CAD build for the part. Positions are in the model's coordinates, mm. A direction names the side the tool comes from. Give positions to 0.01 mm unless a question says otherwise; leave off trailing zeros. Loops run counter-clockwise (first coordinate to the right, second up) from the corner with the lowest first, then second, coordinate; pieces in that order, holes last. Notation, with made-up numbers: (-40, 48.5) -> (10, 48.5) arc R22 cw to (10, 66.5) -> close; hole circle Ø2 at (14, 56). An arc over 180 degrees is marked (long way). Use one line per item in the form item = value.
```python
from build123d import *

# Parameters (mm, degrees)
F0_R      = 15
F1_DEPTH  = 125
F2_W      = 15
F2_H      = 15
F3_ANGLE  = 90
F5_W      = 15
F5_H      = 15
F6_DEPTH  = 75
F8_R      = 5
F9_DEPTH  = 122.5
F10_R     = 5
F11_DEPTH = 122.5


with BuildPart() as f1:
    # F0 (on Right) → F1 (new body, symmetric)
    with BuildSketch(Plane.YZ):
        Circle(F0_R)
    extrude(amount=F1_DEPTH, both=True)

    # F4: F3 across plane


with BuildPart() as f3:
    # F2 (on face) → F3 (revolve)
    with BuildSketch(Plane.YZ.offset(125)):
        Rectangle(F2_W, F2_H)
    revolve(axis=Axis((125, 7.5, 0), (0, 0, 1)), revolution_arc=F3_ANGLE)


with BuildPart() as f1_1:
    add(f1.part)
    add(f3.part.mirror(Plane.YZ))


    add(f3.part)  # F6 merges F3
    # F5 (on face) → F6 (join)
    with BuildSketch(Plane(origin=(0, 7.5, 0), x_dir=(-1, 0, 0), z_dir=(0, 1, 0))):
        with Locations((-132.5, 0)):
            Rectangle(F5_W, F5_H)
    extrude(amount=F6_DEPTH)

    # F7: F1 across plane


with BuildPart() as f1_2:
    add(f1_1.part)
    add(f1_1.part.mirror(Plane.YZ))

    # F8 (on face) → F9 (join)
    with BuildSketch(Plane(origin=(-140, 0, 0), x_dir=(0, -1, 0), z_dir=(-1, 0, 0))):
        with Locations((-70, 0)):
            Circle(F8_R)
    extrude(amount=-F9_DEPTH)

    # F10 (on face) → F11 (join)
    with BuildSketch(Plane.YZ.offset(140)):
        with Locations((70, 0)):
            Circle(F10_R)
    extrude(amount=-F11_DEPTH)


solid = f1_2.part
```
1. Cut at D-D, the plane y = 70. Write the cut outline in (x, z).
Result sheet:
outline = (-140, -7.5) -> (-125, -7.5) -> (-125, -5) -> (-17.5, -5) -> (-17.5, 5) -> (-125, 5) -> (-125, 7.5) -> (-140, 7.5) -> close; (17.5, -5) -> (125, -5) -> (125, -7.5) -> (140, -7.5) -> (140, 7.5) -> (125, 7.5) -> (125, 5) -> (17.5, 5) -> close
2. Drop flat-ended pins along their axis: P1, Ø3, axis at x = 62.5, y = 9.5, coming from the -Z side; P2, Ø2, axis at x = -99, z = 10, coming from the -Y side; P3, Ø12, axis at x = 73.5, z = 5.5, coming from the +Y side. Give the stop position or say it passes through.
Result sheet:
P1 = -12.69
P2 = -12
P3 = 75
3. Tool access for faces 1 (the flat face through (17.5, 70, 0)), 2 (the flat face through (133, 37, -7.5)), 3 (the flat face through (-133, 37, 7.5)), 4 (the cylindrical face through (-72.002, 65.381, -1.915)): list every direction of +Z, -Z, +X, -X, +Y, -Y with a clear straight run to the whole face (end or side of a thin tool).
Result sheet:
face_1 = +Z, -Z, +Y
face_2 = -Z, +X, +Y, -Y
face_3 = +Z, -X, +Y, -Y
face_4 = none
4. Cut at A-A, the plane y = 33.5. Write the cut outline in (x, z), then the cut area to 3 significant figures.
Result sheet:
outline = (-140, -7.5) -> (-125, -7.5) -> (-125, 7.5) -> (-140, 7.5) -> close; (125, -7.5) -> (140, -7.5) -> (140, 7.5) -> (125, 7.5) -> close
area = 450 mm^2
5. Drill centre lines: line 1 (X direction, y = 70, z = -2); line 2 (X direction, y = 28.5, z = 0.25); line 3 (Y direction, x = -89.5, z = -2). Where is each one in solid material? Low to high.
Result sheet:
line_1 = -140 to -17.5, 17.5 to 140
line_2 = -140 to -125, 125 to 140
line_3 = -14.87 to 14.87, 65.42 to 74.58
6. Mould opens along X. For faces 5 (the cylindrical face through (72.002, 74.619, -1.915)), 6 (the flat face through (-133, 37, -7.5)), 7 (the flat face through (-125, -11, 0)) say: pulls with the +X half, pulls with the -X half, needs draft (parallel to the pull), parting line crosses it, or undercut.
Result sheet:
face_5 = undercut
face_6 = needs draft
face_7 = pulls with the -X half
7. Cut at C-C, the plane x = -113.5. Write the cut outline in (y, z), then the cut area to 3 significant figures.
Result sheet:
outline = circle Ø30 at (0, 0); circle Ø10 at (70, 0)
area = 785 mm^2
8. Cut at B-B, the plane z = 0. Write the cut outline in (x, y), then the cut area to 3 significant figures.
Result sheet:
outline = (-140, 7.5) arc R15 ccw to (-125, -7.5) -> (-125, -15) -> (125, -15) -> (125, -7.5) arc R15 ccw to (140, 7.5) -> (140, 82.5) -> (125, 82.5) -> (125, 75) -> (17.5, 75) -> (17.5, 65) -> (125, 65) -> (125, 15) -> (-125, 15) -> (-125, 65) -> (-17.5, 65) -> (-17.5, 75) -> (-125, 75) -> (-125, 82.5) -> (-140, 82.5) -> close
area = 12,300 mm^2
